Could you check a few things on this model? Use its own coordinates, in mm. Round coordinates to 2 decimals unless told otherwise and drop trailing zeros. Order: outer loops, then holes, each group sorted by start corner. A loop starts at its lowest first (then second) coordinate and runs counter-clockwise, first axis right, second up. Notation, with made-up numbers: (85, -24) -> (102, -24) arc R21 ccw to (102, -17) -> close; hole circle Ø4 at (18.25, 70.5). An arc over 180 degrees is marked (long way). One line per question, with ' | ' between items.
```python
from build123d import *

# Parameters (mm, degrees)
F3_R     = 3.683
F4_DEPTH = 25.4
F5_R     = 6.35
F6_DEPTH = 25.4


with BuildPart() as f2:
    # F2: sweep along a path in F0
    with BuildLine(Plane.XZ) as f2_path:
        Line((0, 0), (0, 29.7579510314))
        ThreePointArc((0, 29.7579510314), (3.8669197484, 49.1982693956), (14.8789755157, 65.6789755157))
        Line((14.8789755157, 65.6789755157), (35.9210244843, 86.7210244843))
        ThreePointArc((35.9210244843, 86.7210244843), (52.4017306044, 97.7330802516), (71.8420489686, 101.6))
        Line((71.8420489686, 101.6), (201.2079510314, 101.6))
        ThreePointArc((201.2079510314, 101.6), (220.6482693956, 97.7330802516), (237.1289755157, 86.7210244843))
        Line((237.1289755157, 86.7210244843), (258.1710244843, 65.6789755157))
        ThreePointArc((258.1710244843, 65.6789755157), (269.1830802516, 49.1982693956), (273.05, 29.7579510314))
        Line((273.05, 29.7579510314), (273.05, 0))
    # F1 (on Top) → F2 (sweep)
    with BuildSketch(Plane.XY):
        with BuildLine():
            ThreePointArc((-9.525, -7.9248), (-9.0563122713, -9.0563122713), (-7.9248, -9.525))
            Line((-7.9248, -9.525), (7.9248, -9.525))
            ThreePointArc((7.9248, -9.525), (9.0563122713, -9.0563122713), (9.525, -7.9248))
            Line((9.525, -7.9248), (9.525, 7.9248))
            ThreePointArc((9.525, 7.9248), (9.0563122713, 9.0563122713), (7.9248, 9.525))
            Line((7.9248, 9.525), (-7.9248, 9.525))
            ThreePointArc((-7.9248, 9.525), (-9.0563122713, 9.0563122713), (-9.525, 7.9248))
            Line((-9.525, 7.9248), (-9.525, -7.9248))
        make_face()
        with BuildLine():
            ThreePointArc((-6.35, 4.7498), (-5.8813122713, 5.8813122713), (-4.7498, 6.35))
            Line((-4.7498, 6.35), (4.7498, 6.35))
            ThreePointArc((4.7498, 6.35), (5.8813122713, 5.8813122713), (6.35, 4.7498))
            Line((6.35, 4.7498), (6.35, -4.7498))
            ThreePointArc((6.35, -4.7498), (5.8813122713, -5.8813122713), (4.7498, -6.35))
            Line((4.7498, -6.35), (-4.7498, -6.35))
            ThreePointArc((-4.7498, -6.35), (-5.8813122713, -5.8813122713), (-6.35, -4.7498))
            Line((-6.35, -4.7498), (-6.35, 4.7498))
        make_face(mode=Mode.SUBTRACT)
    sweep(path=f2_path.line)

    # F3 (on Front) → F4 (cut)
    with BuildSketch(Plane.XZ):
        with Locations((0, 16.383)):
            Circle(F3_R)
        with Locations((273.05, 16.383)):
            Circle(F3_R)
    extrude(amount=-F4_DEPTH, mode=Mode.SUBTRACT)

    # F5 (on Front) → F6 (cut)
    with BuildSketch(Plane.XZ):
        with Locations((273.05, 16.383)):
            Circle(F5_R)
        with Locations((0, 16.383)):
            Circle(F5_R)
    extrude(amount=F6_DEPTH, mode=Mode.SUBTRACT)


solid = f2.part
```
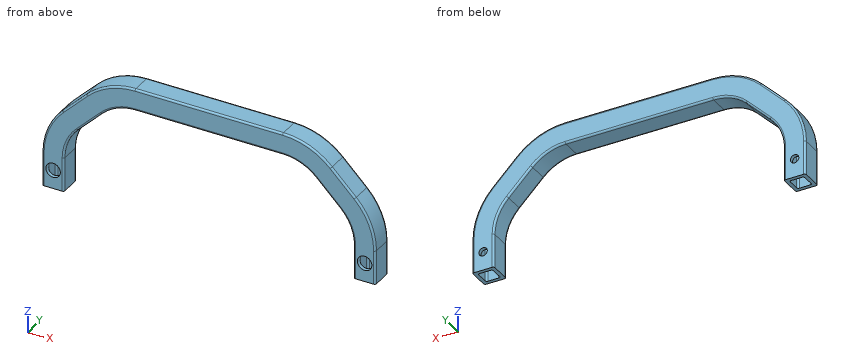
1. I'm going to push flat-ended pins straight in: pin 1 (10 mm diameter, centred on x = 40.5, y = 5, fed in from -Z); pin 2 (3 mm diameter, centred on y = 2.5, z = 68.5, fed in from +X); pin 3 (5 mm diameter, centred on x = 127.5, y = -0.5, fed in from -Z) (3 decimals); pin 4 (9.5 mm diameter, centred on x = 0, z = 16.383, fed in from +Y) (3 decimals). Where does each tip first touch, or does it pass through?
From the geometry:
pin 1: stops at z = 72.83 | pin 2: stops at x = 269.71 | pin 3: stops at z = 92.075 | pin 4: stops at y = 9.525
2. I want a section at A-A on x = 159. List the corners of the cut face in (y, z) for me (3 decimals).
From the geometry:
outline: (-9.525, 93.675) arc R1.6 ccw to (-7.925, 92.075) -> (7.925, 92.075) arc R1.6 ccw to (9.525, 93.675) -> (9.525, 109.525) arc R1.6 ccw to (7.925, 111.125) -> (-7.925, 111.125) arc R1.6 ccw to (-9.525, 109.525) -> close; hole (-6.35, 96.85) arc R1.6 ccw to (-4.75, 95.25) -> (4.75, 95.25) arc R1.6 ccw to (6.35, 96.85) -> (6.35, 106.35) arc R1.6 ccw to (4.75, 107.95) -> (-4.75, 107.95) arc R1.6 ccw to (-6.35, 106.35) -> close
3. I want a section at B-B on x = 273.05. Count the separate pieces of the cut face and the enclosed holes in it, and give its area (3 significant figures).
From the geometry:
separate pieces: 3 | enclosed holes: 0 | area: 413 mm²
4. I need wall thicknesses on probe 1 along Z at (x, y) = (0, 7.2); probe 2 along Z at (x, y) = (168.5, 3.75) (3 decimals); probe 3 along X at (y, z) = (3.75, 46.5). Which ranges of each line are inside material? Lowest first, please.
From the geometry:
probe 1: z = 0 to 12.7, 20.07 to 62.29 | probe 2: z = 92.075 to 95.25, 107.95 to 111.125 | probe 3: x = -7.16 to -3.84, 9.62 to 13.07, 259.98 to 263.43, 276.89 to 280.21
